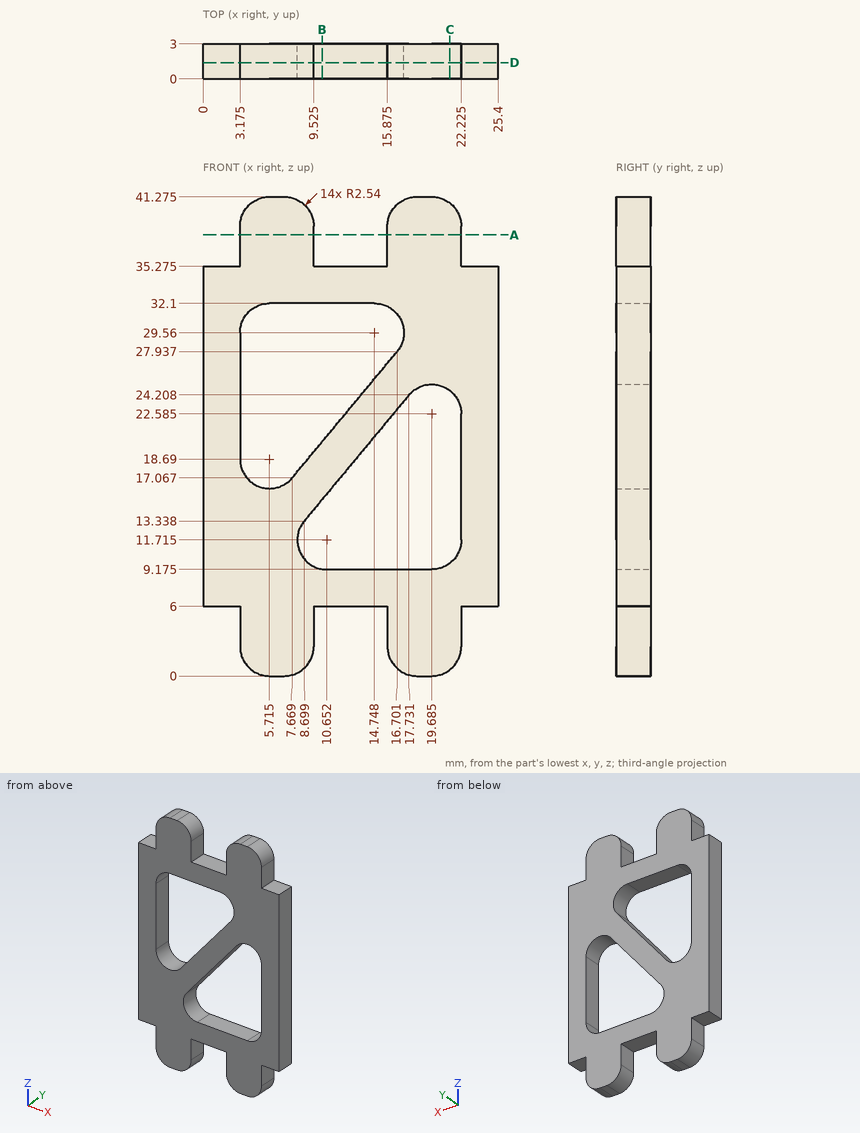
Could you check a few things on this drawing? It's one solid part, dimensions in mm from its lowest x, y, z. Round coordinates to 2 decimals unless told otherwise and drop trailing zeros. Order: outer loops, then holes, each group sorted by start corner. A loop starts at its lowest first (then second) coordinate and runs counter-clockwise, first axis right, second up. Notation, with made-up numbers: (13, 16.25) -> (67, 16.25) arc R20 cw to (67, 32.25) -> close; hole circle Ø10 at (52, -12.75). An arc over 180 degrees is marked (long way). One line per question, with ' | ' between items.
Q1. If we section it at A-A on z = 38: Write out the boundary of the cut face in (x, y) (1 decimal).
Computed values:
outline: (3.2, 0) -> (9.5, 0) -> (9.5, 3) -> (3.2, 3) -> close; (15.9, 0) -> (22.2, 0) -> (22.2, 3) -> (15.9, 3) -> close
Q2. If we section it at D-D on y = 1.4: Give the number of separate pieces and of enclosed holes in the cut face.
Computed values:
separate pieces: 1 | enclosed holes: 2
Q3. If we section it at B-B on x = 10.25: Write out the boundary of the cut face in (y, z) (1 decimal).
Computed values:
outline: (0, 6) -> (3, 6) -> (3, 9.2) -> (0, 9.2) -> close; (0, 15.2) -> (3, 15.2) -> (3, 20.2) -> (0, 20.2) -> close; (0, 32.1) -> (3, 32.1) -> (3, 35.3) -> (0, 35.3) -> close
Q4. I'm going to push flat-ended pins straight in: pin 1 (1.5 mm diameter, centred on x = 12.5, y = 2, fed in from -Z); pin 2 (1.5 mm diameter, centred on y = 2, z = 38, fed in from -X) (1 decimal); pin 3 (1.5 mm diameter, centred on x = 13, y = 1, fed in from +Z) (1 decimal). Where does each tip first touch, or does it pass through?
Computed values:
pin 1: z = 6 | pin 2: x = 3.2 | pin 3: z = 35.3
Q5. If we section it at C-C on x = 21.25: Write out the boundary of the cut face in (y, z) (1 decimal).
Computed values:
outline: (0, 0.5) -> (3, 0.5) -> (3, 9.7) -> (0, 9.7) -> close; (0, 24.6) -> (3, 24.6) -> (3, 40.7) -> (0, 40.7) -> close
Q6. If I drill on line 1 (X direction, y = 0.25, z = 29.5) (1 decimal); line 2 (Z direction, x = 8.5, y = 0.7) (1 decimal); line 3 (X direction, y = 1.15, z = 18) (1 decimal), over which ranges is the centre line in solid material (lowest first)? Write a range as from..to.
Computed values:
line 1: 0..3.2, 17.3..25.4 | line 2: 0.5..10.4, 13.1..18.1, 32.1..40.8 | line 3: 0..3.3, 8.4..12.6, 22.2..25.4
